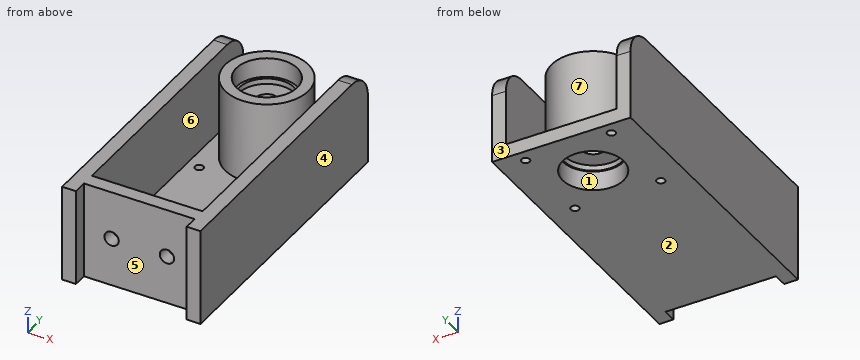
from build123d import *

# Parameters (mm, degrees)
SKETCH_W        = 50
SKETCH_H        = 100
SKETCH_R        = 11
PAD_DEPTH       = 5
PAD001_DEPTH    = 5
PAD002_DEPTH    = 5
SKETCH003_W     = 40
SKETCH003_H     = 5
PAD003_DEPTH    = 30
SKETCH004_R     = 1.5
POCKET_DEPTH    = 5
SKETCH005_R     = 15
PAD004_DEPTH    = 30
SKETCH006_R     = 11
POCKET001_DEPTH = 7
SKETCH007_R     = 10
POCKET002_DEPTH = 2
SKETCH008_R     = 4.25
POCKET003_DEPTH = 26.001
SKETCH009_R     = 11
POCKET004_DEPTH = 2
SKETCH010_R     = 10.5
POCKET005_DEPTH = 2
SKETCH011_R     = 2.6
POCKET006_DEPTH = 5
FILLET_R        = 10


with BuildPart() as part:
    # Sketch → Pad (new body)
    with BuildSketch(Plane.XY):
        Rectangle(SKETCH_W, SKETCH_H)
        with Locations((0, 30)):
            Circle(SKETCH_R, mode=Mode.SUBTRACT)
    extrude(amount=PAD_DEPTH)

    # Sketch001 (on Face1 of Pad) → Pad001 (join)
    with BuildSketch(Plane(origin=(-25, 0, 0), x_dir=(0, -1, 0), z_dir=(-1, 0, 0))):
        Polygon((-50, 5), (-50, 35), (55, 35), (55, 0), (50, 0), (50, 5), align=None)
    extrude(amount=-PAD001_DEPTH)

    # Sketch002 (on Face4 of Pad001) → Pad002 (join)
    with BuildSketch(Plane.YZ.offset(25)):
        Polygon((-50, 0), (-55, 0), (-55, 35), (50, 35), (50, 5), (-50, 5), align=None)
    extrude(amount=-PAD002_DEPTH)

    # Sketch003 (on Face7 of Pad002) → Pad003 (join)
    with BuildSketch(Plane.XY.offset(5)):
        with Locations((0, -47.5)):
            Rectangle(SKETCH003_W, SKETCH003_H)
    extrude(amount=PAD003_DEPTH)

    # Sketch004 (on Face9 of Pad003) → Pocket (cut)
    with BuildSketch(Plane.XY.offset(5)):
        with Locations((-15.5, 45.5)):
            Circle(SKETCH004_R)
        with Locations((-15.5, 14.5)):
            Circle(SKETCH004_R)
        with Locations((15.5, 14.5)):
            Circle(SKETCH004_R)
        with Locations((15.5, 45.5)):
            Circle(SKETCH004_R)
    extrude(amount=-POCKET_DEPTH, mode=Mode.SUBTRACT)

    # Sketch005 (on Face6 of Pocket) → Pad004 (join)
    with BuildSketch(Plane.XY.offset(5)):
        with Locations((0, 30)):
            Circle(SKETCH005_R)
    extrude(amount=PAD004_DEPTH)

    # Sketch006 (on Face22 of Pad004) → Pocket001 (cut)
    with BuildSketch(Plane.XY.offset(35)):
        with Locations((0, 30)):
            Circle(SKETCH006_R)
    extrude(amount=-POCKET001_DEPTH, mode=Mode.SUBTRACT)

    # Sketch007 (on Face24 of Pocket001) → Pocket002 (cut)
    with BuildSketch(Plane.XY.offset(28)):
        with Locations((0, 30)):
            Circle(SKETCH007_R)
    extrude(amount=-POCKET002_DEPTH, mode=Mode.SUBTRACT)

    # Sketch008 (on Face26 of Pocket002) → Pocket003 (cut, through all)
    with BuildSketch(Plane.XY.offset(26)):
        with Locations((0, 30)):
            Circle(SKETCH008_R)
    extrude(amount=-POCKET003_DEPTH, mode=Mode.SUBTRACT)

    # Sketch009 (on Face21 of Pocket003) → Pocket004 (cut)
    with BuildSketch(Plane(origin=(0, 0, 5), x_dir=(1, 0, 0), z_dir=(0, 0, -1))):
        with Locations((0, -30)):
            Circle(SKETCH009_R)
    extrude(amount=-POCKET004_DEPTH, mode=Mode.SUBTRACT)

    # Sketch010 (on Face24 of Pocket004) → Pocket005 (cut)
    with BuildSketch(Plane(origin=(0, 0, 7), x_dir=(1, 0, 0), z_dir=(0, 0, -1))):
        with Locations((0, -30)):
            Circle(SKETCH010_R)
    extrude(amount=-POCKET005_DEPTH, mode=Mode.SUBTRACT)

    # Sketch011 (on Face12 of Pocket005) → Pocket006 (cut)
    with BuildSketch(Plane.XZ.offset(50)):
        with Locations((-10, 17.5)):
            Circle(SKETCH011_R)
        with Locations((10, 17.5)):
            Circle(SKETCH011_R)
    extrude(amount=-POCKET006_DEPTH, mode=Mode.SUBTRACT)

    # Fillet
    fillet_edges = [part.edges().sort_by_distance(p)[0] for p in [
        (22.5, 50, 35),
        (-22.5, 50, 35),
    ]]
    fillet(fillet_edges, radius=FILLET_R)


solid = part.part
Here's how the part is built. I have some questions about the finished solid (model axes, mm). Face numbers are marked on the shaded views. A direction names the side the tool comes from. Coordinates: 2 decimals unless noted, no trailing zeros. Write each loop counter-clockwise with the first axis right and the second up, starting at its lowest first coordinate (ties: lowest second). Pieces come first, ordered by that corner, then holes.
Item 1: On a 3-axis mill with a long thin cutter (end or side, diameter ignored), from which of +Z, -Z, +X, -X, +Y, -Y can I reach the whole of each face in a straight line? I mean the marked faces 4, 5, 6 and 7. Say none if no direction works.
Item 2: I want a section at B-B on z = 17.5. Write out the boundary of the cut face in (x, y).
Item 3: Will these pins go through, and if not, where does the flat tip stop? pin 1 (13 mm diameter, centred on x = 0, y = 30, fed in from -Z); pin 2 (4 mm diameter, centred on x = -10, z = 17.5, fed in from -Y); pin 3 (4 mm diameter, centred on x = 11.5, y = -39.5, fed in from -Z); pin 4 (6 mm diameter, centred on x = -7, y = 33.5, fed in from +Z).
Item 4: If we mould it in two halves opening along Y, with no side actions, what happens to the marked faces 1, 2 and 3? For each: +Y half, -Y half, draft (parallel to the pull), parting line (faces both ways), or undercut.
Item 5: If I drill on line 1 (Y direction, x = 0, z = 32.25); line 2 (Z direction, x = 10, y = -48); line 3 (Y direction, x = -15, z = 2), over which ranges is the centre line in solid material (lowest first)?
Item 6: I want a section at A-A on z = 13. Write out the boundary of the cut face in (x, y).
Findings below:
1. face 4: +Z, -Z, +X, +Y, -Y
1. face 5: +Z, -Z, -Y
1. face 6: +Z, +Y
1. face 7: +Z
2. outline: (-25, -55) - (-20, -55) - (-20, -50) - (-12.6, -50) - (-12.6, -45) - (-20, -45) - (-20, 50) - (-25, 50) - close; circle Ø30 at (0, 30); (-7.4, -50) - (7.4, -50) - (7.4, -45) - (-7.4, -45) - close; (12.6, -50) - (20, -50) - (20, -55) - (25, -55) - (25, 50) - (20, 50) - (20, -45) - (12.6, -45) - close; hole circle Ø8.5 at (0, 30)
3. pin 1: stops at z = 9
3. pin 2: stops at y = 17.31
3. pin 3: stops at z = 0
3. pin 4: stops at z = 28
4. face 1: undercut
4. face 2: draft
4. face 3: +Y half
5. line 1: y = -50 to -45, 15 to 19, 41 to 45
5. line 2: z = 0 to 14.9, 20.1 to 35
5. line 3: y = -50 to 13.09, 15.91 to 44.09, 46.91 to 50
6. outline: (-25, -55) - (-20, -55) - (-20, -50) - (20, -50) - (20, -55) - (25, -55) - (25, 50) - (20, 50) - (20, -45) - (-20, -45) - (-20, 50) - (-25, 50) - close; circle Ø30 at (0, 30); hole circle Ø8.5 at (0, 30)
